Source: CAD feature listing. Evaluate the final solid. Frame: model axes, mm. Face numbers are marked on the shaded views. A direction names the side the tool comes from. Round coordinates to 2 decimals unless told otherwise and drop trailing zeros. Loops run counter-clockwise (first coordinate to the right, second up) from the corner with the lowest first, then second, coordinate; pieces in that order, holes last. Notation, with made-up numbers: (-34, 74) - (22, 74) arc R29 ccw to (22, 97) - close; hole circle Ø10 at (3, 56). An arc over 180 degrees is marked (long way). One line per question, with ' | ' between items.
from build123d import *

# Parameters (mm, degrees)
EXTRUDE_1_DEPTH     = 48
SKETCH_3_R          = 4.25
CUT_EXTRUDE_1_DEPTH = 82.043198357


with BuildPart() as part:
    # 草图1 → 凸台-拉伸1 (new, symmetric)
    with BuildSketch(Plane.XY):
        Polygon((0, 0), (50, 0), (50, 50), (42, 50), (42, 29.242640687), (20.757359313, 8), (0, 8), align=None)
        with BuildLine():
            Line((37.061279898, 14.352933665), (35.340960992, 16.07325257))
            ThreePointArc((35.340960992, 16.07325257), (39.856939547, 16.192314452), (42.15, 12.3))
            Line((42.15, 12.3), (45, 12.3))
            Line((45, 12.3), (45, 23.171572875))
            ThreePointArc((45, 23.171572875), (43.765366865, 25.01933194), (41.585786438, 24.585786438))
            Line((41.585786438, 24.585786438), (25.414213562, 8.414213562))
            ThreePointArc((25.414213562, 8.414213562), (24.98066806, 6.234633135), (26.828427125, 5))
            Line((26.828427125, 5), (37.7, 5))
            Line((37.7, 5), (37.7, 7.85))
            ThreePointArc((37.7, 7.85), (33.807685548, 10.143060453), (33.92674743, 14.659039008))
            Line((33.92674743, 14.659039008), (35.647066335, 12.938720102))
            ThreePointArc((35.647066335, 12.938720102), (39.22027958, 10.77972042), (37.061279898, 14.352933665))
        make_face(mode=Mode.SUBTRACT)
    extrude(amount=EXTRUDE_1_DEPTH, both=True)

    # 草图3 → 切除-拉伸1 (cut, through all)
    with BuildSketch(Plane(origin=(0, 8, 0), x_dir=(1, 0, 0), z_dir=(0, 1, 0))):
        with Locations(Location((10, 25, 0), (0, 0, 270))):
            Circle(SKETCH_3_R)
        with Locations(Location((10, -25, 0), (0, 0, 90))):
            Circle(SKETCH_3_R)
    cut_extrude_1 = extrude(amount=-CUT_EXTRUDE_1_DEPTH, mode=Mode.SUBTRACT)

    # 镜向1: 切除-拉伸1 across plane
    add(cut_extrude_1.mirror(Plane(origin=(25, 25, 0), x_dir=(0, 0, 1), z_dir=(-0.7071067811865486, -0.7071067811865465, 0))), mode=Mode.SUBTRACT)


solid = part.part
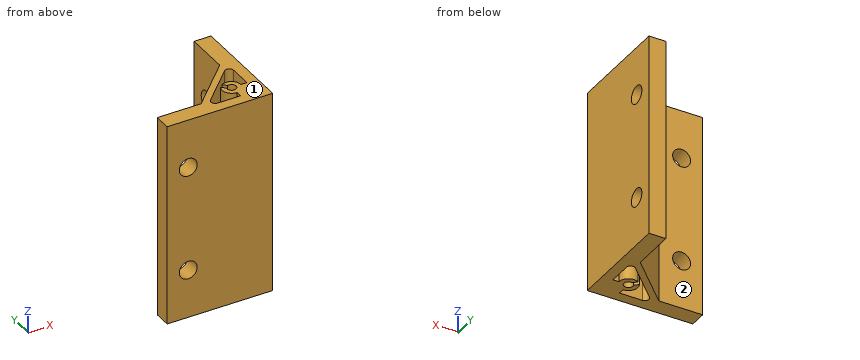
1. Section query D-D, the plane x = 32. Return loops of the section in (y, z), plus the area to 3 significant figures.
Worked out:
outline: (0, -48) - (5, -48) - (5, 48) - (0, 48) - close; (15, -48) - (19.24, -48) - (19.24, 48) - (15, 48) - close | area: 887 mm2
2. Section query B-B, the plane y = 38. Return loops of the section in (x, z).
Worked out:
outline: (42, -48) - (50, -48) - (50, -28.75) - (42, -28.75) - close; (42, -21.25) - (50, -21.25) - (50, 21.25) - (42, 21.25) - close; (42, 28.75) - (50, 28.75) - (50, 48) - (42, 48) - close
3. Contact query for flat-ended pins moving along their axis: P1, Ø3, axis at x = 38.5, y = 28, coming from the -Z side; P2, Ø12, axis at y = 16.5, z = 18.5, coming from the -X side; P3, Ø23, axis at y = 44.5, z = 1.5, coming from the -X side; P4, Ø12, axis at x = 32, z = -11.5, coming from the +Y side. Output: stop coordinate, or through.
Worked out:
P1: passes through | P2: stops at x = 23.26 | P3: stops at x = 42 | P4: stops at y = 25.24
4. Access query for the marked faces 1 and 2. Directions: +Z, -Z, +X, -X, +Y, -Y. A direction counts if a zero-diameter tool reaches every point of the face in a straight line with its end or side. Return the directions, or none.
Worked out:
face 1: +Z, +X, -X, +Y, -Y | face 2: +Z, -Z, -X, +Y
5. Material intervals for probe 1 along Z at (x, y) = (43, 40); probe 2 along Y at (x, z) = (39, 28.5); probe 3 along X at (y, z) = (14, 29), sorted ascending.
Worked out:
probe 1: z = -48 to -29.25, -20.75 to 20.75, 29.25 to 48 | probe 2: y = 0 to 10.59, 14.01 to 16.56, 22 to 26.24 | probe 3: x = 26.76 to 31, 33.59 to 34.59, 39.02 to 41.81, 45 to 50
6. Section query C-C, the plane z = -4.5. Return loops of the section in (x, y).
Worked out:
outline: (0, 0) - (50, 0) - (50, 50) - (42, 50) - (42, 29.24) - (20.76, 8) - (0, 8) - close; hole (25.41, 8.41) arc R2 ccw to (26.83, 5) - (37.7, 5) - (37.7, 7.85) arc R4.45 cw to (33.93, 14.66) - (35.65, 12.94) arc R2.15 ccw (long way) to (37.06, 14.35) - (35.34, 16.07) arc R4.45 cw to (42.15, 12.3) - (45, 12.3) - (45, 23.17) arc R2 ccw to (41.59, 24.59) - close
7. Section query A-A, the plane z = 25. Return loops of the section in (x, y).
Worked out:
outline: (0, 0) - (5.75, 0) - (5.75, 8) - (0, 8) - close; (14.25, 0) - (50, 0) - (50, 35.75) - (42, 35.75) - (42, 29.24) - (20.76, 8) - (14.25, 8) - close; (42, 44.25) - (50, 44.25) - (50, 50) - (42, 50) - close; hole (25.41, 8.41) arc R2 ccw to (26.83, 5) - (37.7, 5) - (37.7, 7.85) arc R4.45 cw to (33.93, 14.66) - (35.65, 12.94) arc R2.15 ccw (long way) to (37.06, 14.35) - (35.34, 16.07) arc R4.45 cw to (42.15, 12.3) - (45, 12.3) - (45, 23.17) arc R2 ccw to (41.59, 24.59) - close
